Here's how the part is built. I have some questions about the finished solid (model axes, mm). Face numbers are marked on the shaded views. A direction names the side the tool comes from. Round coordinates to 2 decimals unless told otherwise and drop trailing zeros. Loops run counter-clockwise (first coordinate to the right, second up) from the corner with the lowest first, then second, coordinate; pieces in that order, holes last. Notation, with made-up numbers: (-7.75, -21.5) -> (18.25, -21.5) arc R27 ccw to (18.25, 16.5) -> close; hole circle Ø11 at (39.25, 51). An arc over 180 degrees is marked (long way). One line per item, written item: value. Start each with the question number.
```python
from build123d import *

# Parameters (mm, degrees)
F0_R     = 17.4625
F0_R_2   = 25.4
F1_DEPTH = 9.525
F2_DEPTH = 25.4
F3_DEPTH = 15.875


with BuildPart() as f1:
    # F0 (on Front) → F1 (new body, symmetric)
    with BuildSketch(Plane.XZ):
        with BuildLine():
            ThreePointArc((-145.4689772406, -33.2912941566), (-120.7699308937, -24.185564488), (-110.3768719775, 0))
            ThreePointArc((-110.3768719775, 0), (-120.7699308937, 24.185564488), (-145.4689772406, 33.2912941566))
            ThreePointArc((-145.4689772406, 33.2912941566), (-177.0518719775, 0), (-145.4689772406, -33.2912941566))
        make_face()
        with Locations((-143.7143719775, 0)):
            Circle(F0_R, mode=Mode.SUBTRACT)
        with BuildLine():
            ThreePointArc((-145.4689772406, 33.2912941566), (-120.7699308937, 24.185564488), (-110.3768719775, 0))
            ThreePointArc((-110.3768719775, 0), (-120.7699308937, -24.185564488), (-145.4689772406, -33.2912941566))
            Line((-145.4689772406, -33.2912941566), (35.0047069699, -42.803092487))
            ThreePointArc((35.0047069699, -42.803092487), (-5.6018719775, 0), (35.0047069699, 42.803092487))
            Line((35.0047069699, 42.803092487), (-145.4689772406, 33.2912941566))
        make_face()
        with BuildLine():
            ThreePointArc((80.1231280225, 0), (66.7606237016, 31.0957257703), (35.0047069699, 42.803092487))
            ThreePointArc((35.0047069699, 42.803092487), (-5.6018719775, 0), (35.0047069699, -42.803092487))
            ThreePointArc((35.0047069699, -42.803092487), (66.7606237016, -31.0957257703), (80.1231280225, 0))
        make_face()
        with Locations((37.2606280225, 0)):
            Circle(F0_R_2, mode=Mode.SUBTRACT)
    extrude(amount=F1_DEPTH, both=True)

    # F0 (on Front) → F2 (join, symmetric)
    with BuildSketch(Plane.XZ):
        with BuildLine():
            ThreePointArc((80.1231280225, 0), (66.7606237016, 31.0957257703), (35.0047069699, 42.803092487))
            ThreePointArc((35.0047069699, 42.803092487), (-5.6018719775, 0), (35.0047069699, -42.803092487))
            ThreePointArc((35.0047069699, -42.803092487), (66.7606237016, -31.0957257703), (80.1231280225, 0))
        make_face()
        with Locations((37.2606280225, 0)):
            Circle(F0_R_2, mode=Mode.SUBTRACT)
    extrude(amount=F2_DEPTH, both=True)

    # F0 (on Front) → F3 (join, symmetric)
    with BuildSketch(Plane.XZ):
        with BuildLine():
            ThreePointArc((-145.4689772406, -33.2912941566), (-120.7699308937, -24.185564488), (-110.3768719775, 0))
            ThreePointArc((-110.3768719775, 0), (-120.7699308937, 24.185564488), (-145.4689772406, 33.2912941566))
            ThreePointArc((-145.4689772406, 33.2912941566), (-177.0518719775, 0), (-145.4689772406, -33.2912941566))
        make_face()
        with Locations((-143.7143719775, 0)):
            Circle(F0_R, mode=Mode.SUBTRACT)
    extrude(amount=F3_DEPTH, both=True)


solid = f1.part
```
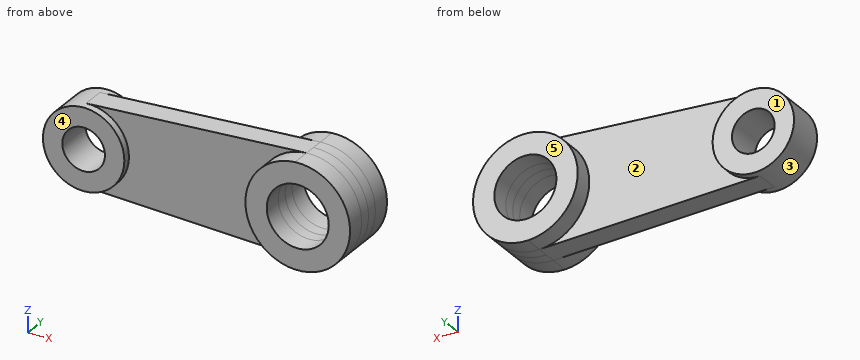
Q1. I want a section at D-D on x = -1.5. Please give me the cut outline in (y, z) (3 decimals).
Q2. I want a section at A-A on z = 0. Please give me the cut outline in (x, y) (3 decimals), plus the area to 3 significant figures.
Q3. If we mould it in two halves opening along X, with no side actions, what happens to the marked faces 1 and 2? For each: released by +X, released by -X, zero draft, split by the parting line, or undercut.
Q4. Will these pins go through, and if not, where does the flat tip stop? P1, Ø5, axis at x = -84.5, z = -27.5, coming from the -Y side (3 decimals); P2, Ø5, axis at x = -2.5, z = 22.5, coming from the +Y side (3 decimals); P3, Ø3, axis at x = 32, y = -9, coming from the -Z side.
Q5. I want a section at C-C on z = -23. Please give me the cut outline in (x, y) (3 decimals), plus the area to 3 significant figures.
Q6. I want a section at B-B on y = 13. Please give me the cut outline in (x, z) (1 decimal).
Q7. If I drill on line 1 along X through (y, z) = (10, -5); line 2 along X through (y, z) = (-14, -2); line 3 along Y through (x, z) = (-79, -3.5) (3 decimals), over which ranges is the centre line in solid material (lowest first)?
Q8. Which directions (+Z, -Z, +X, -X, +Y, -Y) give clear straight access to the entire face, cutting with the end or side of a thin tool? Please do the marked faces 3, 4 and 5.
Answers below:
1. outline: (-25.4, -18.298) -> (-9.525, -18.298) -> (-9.525, -40.879) -> (9.525, -40.879) -> (9.525, -18.298) -> (25.4, -18.298) -> (25.4, 18.298) -> (9.525, 18.298) -> (9.525, 40.879) -> (-9.525, 40.879) -> (-9.525, 18.298) -> (-25.4, 18.298) -> close
2. outline: (-177.052, -15.875) -> (-161.177, -15.875) -> (-161.177, 15.875) -> (-177.052, 15.875) -> close; (-126.252, -15.875) -> (-110.377, -15.875) -> (-110.377, -9.525) -> (-5.602, -9.525) -> (-5.602, -25.4) -> (11.861, -25.4) -> (11.861, 25.4) -> (-5.602, 25.4) -> (-5.602, 9.525) -> (-110.377, 9.525) -> (-110.377, 15.875) -> (-126.252, 15.875) -> close; (62.661, -25.4) -> (80.123, -25.4) -> (80.123, 25.4) -> (62.661, 25.4) -> close
2. area: 4,780 mm^2
3. face 1: zero draft
3. face 2: undercut
4. P1: stops at y = -9.525
4. P2: stops at y = 9.525
4. P3: stops at z = -42.72
5. outline: (-167.847, -15.875) -> (-119.582, -15.875) -> (-119.582, -9.525) -> (1.092, -9.525) -> (1.092, -25.4) -> (26.483, -25.4) -> (26.483, 25.4) -> (1.092, 25.4) -> (1.092, 9.525) -> (-119.582, 9.525) -> (-119.582, 15.875) -> (-167.847, 15.875) -> close; (48.038, -25.4) -> (73.43, -25.4) -> (73.43, 25.4) -> (48.038, 25.4) -> close
5. area: 6,410 mm^2
6. outline: circle Ø66.7 at (-143.7, 0); circle Ø85.7 at (37.3, 0); hole circle Ø34.9 at (-143.7, 0); hole circle Ø50.8 at (37.3, 0)
7. line 1: x = -176.67 to -160.45, -126.98 to -110.75, -5.31 to 12.36, 62.16 to 79.83
7. line 2: x = -176.99 to -161.06, -126.37 to -110.44, -5.56 to 11.94, 62.58 to 80.08
7. line 3: y = -9.525 to 9.525
8. face 3: none
8. face 4: +Z, -Z, -X, -Y
8. face 5: +Z, -Z, +X, -X, +Y
